Answer from the drawing. Dimensions are ordinates in mm from the lowest x, y and z of the part. A direction names the side the tool comes from. Round coordinates to 2 decimals unless told otherwise and drop trailing zeros. Loops run counter-clockwise (first coordinate to the right, second up) from the corner with the lowest first, then second, coordinate; pieces in that order, holes last.
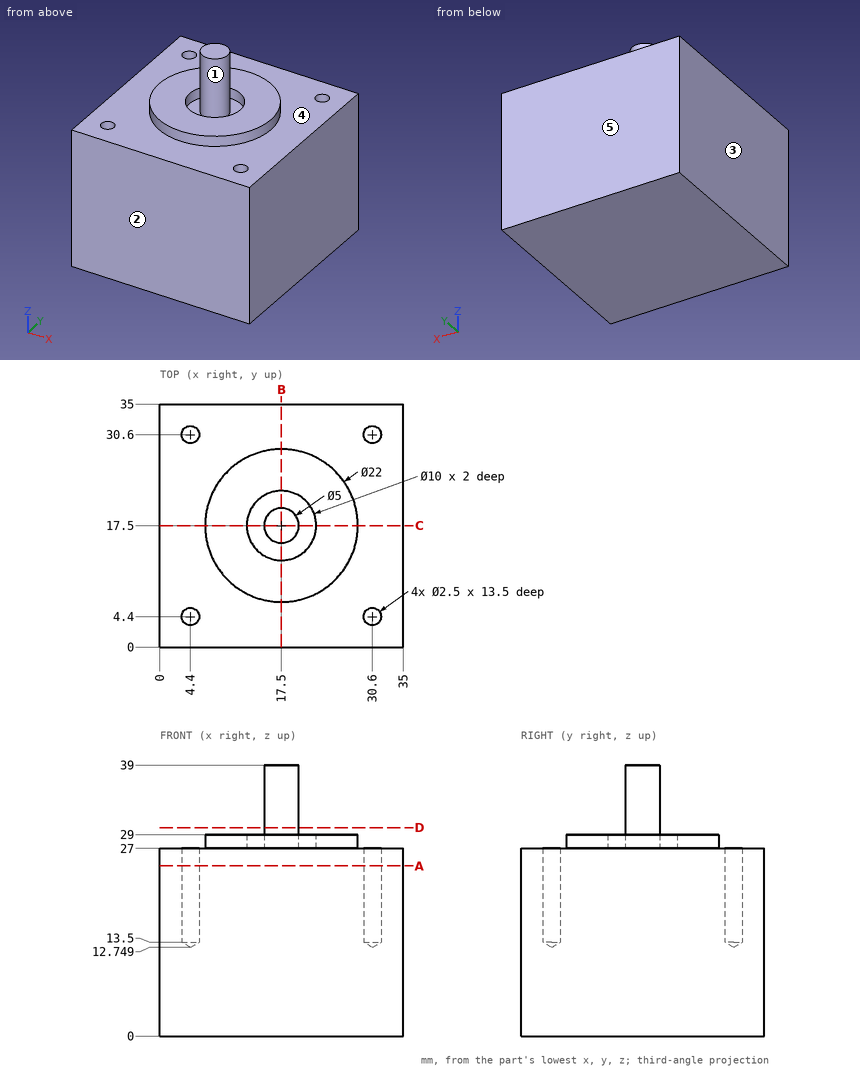
Item 1: Determine the mould class of the marked faces 1, 2 and 3 for opening direction X: pulls with the +X half, pulls with the -X half, needs draft (parallel to the pull), parting line crosses it, or undercut.
Item 2: For the marked faces 4 and 5, determine the directions among +Z, -Z, +X, -X, +Y, -Y from which every point of the face is accessible in a straight line to the end or side of a thin tool.
Item 3: Section B-B, the plane x = 17.5 is taken. Give the vertices of the cut face in (y, z).
Item 4: Section D-D, the plane z = 30 is taken. Give the vertices of the cut face in (x, y).
Item 5: Section A-A, the plane z = 24.5 is taken. Give the vertices of the cut face in (x, y), plus the area to 3 significant figures.
Item 6: Straight lines are drawn through the part: line 1 (X direction, y = 30.6, z = 20.75); line 2 (X direction, y = 30, z = 16). For each, find the intervals that lie inside material, in ascending order.
Item 7: Each of these flat-tipped pins is pushed along its axis until it touches: P1, Ø5, axis at x = 17.5, y = 4.5, coming from the +Z side; P2, Ø2, axis at x = 30.6, y = 4.4, coming from the +Z side. Where does it stop, or does it pass through?
Answer below:
1. face 1: undercut
1. face 2: needs draft
1. face 3: pulls with the -X half
2. face 4: +Z
2. face 5: +Z, -Z, +X, -X, +Y
3. outline: (0, 0) - (35, 0) - (35, 27) - (28.5, 27) - (28.5, 29) - (22.5, 29) - (22.5, 27) - (20, 27) - (20, 39) - (15, 39) - (15, 27) - (12.5, 27) - (12.5, 29) - (6.5, 29) - (6.5, 27) - (0, 27) - close
4. outline: circle Ø5 at (17.5, 17.5)
5. outline: (0, 0) - (35, 0) - (35, 35) - (0, 35) - close; hole circle Ø2.5 at (4.4, 4.4); hole circle Ø2.5 at (4.4, 30.6); hole circle Ø2.5 at (30.6, 4.4); hole circle Ø2.5 at (30.6, 30.6)
5. area: 1,210 mm2
6. line 1: x = 0 to 3.15, 5.65 to 29.35, 31.85 to 35
6. line 2: x = 0 to 3.3, 5.5 to 29.5, 31.7 to 35
7. P1: stops at z = 29
7. P2: stops at z = 13.35
